```python
from build123d import *

# Parameters (mm, degrees)
SKETCH_W        = 75
SKETCH_H        = 55
PAD_DEPTH       = 3
SKETCH001_W     = 75
SKETCH001_H     = 55
SKETCH001_W_2   = 71
SKETCH001_H_2   = 51
PAD001_DEPTH    = 10
SKETCH002_W     = 5
SKETCH002_H     = 5
PAD002_DEPTH    = 5
SKETCH011_R     = 0.6
POCKET004_DEPTH = 5
SKETCH012_W     = 56
SKETCH012_H     = 10
PAD003_DEPTH    = 4
SKETCH013_W     = 8
SKETCH013_H     = 5
POCKET_DEPTH    = 8
SKETCH014_W     = 75
SKETCH014_H     = 8
PAD004_DEPTH    = 30
SKETCH015_R     = 6
PAD005_DEPTH    = 10
SKETCH016_R     = 6
PAD006_DEPTH    = 10
SKETCH017_R     = 2.2
POCKET005_DEPTH = 75
SKETCH018_W     = 55
SKETCH018_H     = 8
POCKET006_DEPTH = 8


with BuildPart() as part:
    # Sketch → Pad (new body)
    with BuildSketch(Plane.XY):
        with Locations((0, 27.5)):
            Rectangle(SKETCH_W, SKETCH_H)
    extrude(amount=PAD_DEPTH)

    # Sketch001 (on Face6 of Pad) → Pad001 (join)
    with BuildSketch(Plane.XY.offset(3)):
        with Locations((0, 27.5)):
            Rectangle(SKETCH001_W, SKETCH001_H)
        with Locations((0, 27.5)):
            Rectangle(SKETCH001_W_2, SKETCH001_H_2, mode=Mode.SUBTRACT)
    extrude(amount=PAD001_DEPTH)

    # Sketch002 (on Face15 of Pad001) → Pad002 (join)
    with BuildSketch(Plane.XY.offset(3)):
        with Locations((-33, 50.5)):
            Rectangle(SKETCH002_W, SKETCH002_H)
        with Locations((33, 50.5)):
            Rectangle(SKETCH002_W, SKETCH002_H)
        with Locations((33, 4.5)):
            Rectangle(SKETCH002_W, SKETCH002_H)
        with Locations((-33, 4.5)):
            Rectangle(SKETCH002_W, SKETCH002_H)
    extrude(amount=PAD002_DEPTH)

    # Sketch011 → Pocket004 (cut)
    with BuildSketch(Plane.XY.offset(8)):
        with Locations((-33, 4.5)):
            Circle(SKETCH011_R)
        with Locations((33, 4.5)):
            Circle(SKETCH011_R)
        with Locations((-33, 50.5)):
            Circle(SKETCH011_R)
        with Locations((33, 50.5)):
            Circle(SKETCH011_R)
    extrude(amount=-POCKET004_DEPTH, mode=Mode.SUBTRACT)

    # Sketch012 (on Face17 of Pocket004) → Pad003 (join)
    with BuildSketch(Plane.XY.offset(3)):
        with Locations((0, 33)):
            Rectangle(SKETCH012_W, SKETCH012_H)
    extrude(amount=PAD003_DEPTH)

    # Sketch013 (on Face37 of Pad003) → Pocket (cut)
    with BuildSketch(Plane.XY.offset(7)):
        with Locations((-19, 33.5)):
            Rectangle(SKETCH013_W, SKETCH013_H)
        with Locations((19, 33.5)):
            Rectangle(SKETCH013_W, SKETCH013_H)
    extrude(amount=-POCKET_DEPTH, mode=Mode.SUBTRACT)

    # Sketch014 (on Face4 of Pocket) → Pad004 (join)
    with BuildSketch(Plane(origin=(0, 0, 0), x_dir=(1, 0, 0), z_dir=(0, 0, -1))):
        with Locations((0, 4)):
            Rectangle(SKETCH014_W, SKETCH014_H)
    extrude(amount=-PAD004_DEPTH)

    # Sketch015 (on Face6 of Pad004) → Pad005 (join)
    with BuildSketch(Plane(origin=(-37.5, 0, 0), x_dir=(0, -1, 0), z_dir=(-1, 0, 0))):
        with Locations((4, 30)):
            Circle(SKETCH015_R)
    extrude(amount=-PAD005_DEPTH)

    # Sketch016 (on Face8 of Pad005) → Pad006 (join)
    with BuildSketch(Plane.YZ.offset(37.5)):
        with Locations((-4, 30)):
            Circle(SKETCH016_R)
    extrude(amount=-PAD006_DEPTH)

    # Sketch017 (on Face37 of Pad006) → Pocket005 (cut)
    with BuildSketch(Plane.YZ.offset(37.5)):
        with Locations((-4, 30)):
            Circle(SKETCH017_R)
    extrude(amount=-POCKET005_DEPTH, mode=Mode.SUBTRACT)

    # Sketch018 (on Face37 of Pocket005) → Pocket006 (cut)
    with BuildSketch(Plane.XY.offset(30)):
        with Locations((0, -4)):
            Rectangle(SKETCH018_W, SKETCH018_H)
    extrude(amount=-POCKET006_DEPTH, mode=Mode.SUBTRACT)


solid = part.part
```
Verification items for the finished model (mm, model axes). A direction names the side the tool comes from. Coordinates: 2 decimals unless noted, no trailing zeros. Write each loop counter-clockwise with the first axis right and the second up, starting at its lowest first coordinate (ties: lowest second). Pieces come first, ordered by that corner, then holes. Notation, with made-up numbers: M -19.5,-19 L -11.5,-19 A16 ccw -11.5,11 Z; hole C 54.5,-26 d5. An arc over 180 degrees is marked long. Answer as a JSON object with one key per item and string values. Group by question number.
(1) Cross-section at D-D, the plane z = 10.5. Record the cut outline in (x, y).
(2) Cross-section at C-C, the plane x = 18.5. Record the cut outline in (y, z), and give its area (3 significant figures).
(3) Cross-section at A-A, the plane z = 4.5. State how many separate pieces and enclosed holes the cut face has, and give its area (3 significant figures).
(4) Material ranges on line 1 (X direction, y = 32.5, z = 6); line 2 (Y direction, x = 13, z = 6); line 3 (Y direction, x = -33, z = 6), recorded low to high.
(5) Tool access check on faces 4 (the face through (-35.5, 27, 8)), 5 (the face through (-15, 33, 4)), 6 (the face through (-27.5, -4.1, 27.5)). Record the directions out of +Z, -Z, +X, -X, +Y, -Y that give a thin tool (end or side, any length) a straight path to the whole face; none if there is none.
(6) Cross-section at B-B, the plane y = -4. Record the cut outline in (x, z).
(7) Release check for a two-part mould opening along Y. For faces 1 (the face through (27.5, -4.1, 27.5)), 2 (the face through (33, -4, 36)), 3 (the face through (0, 28, 5)) record: +Y half, -Y half, draft (parallel to the pull), parting line (faces both ways), or undercut.
(8) Gauge pin test, flat ends, axial feed: pin 1 (6 mm diameter, centred on y = -4.5, z = 30, fed in from -X); pin 2 (2 mm diameter, centred on x = -20, z = 2, fed in from -Y); pin 3 (0.6 mm diameter, centred on x = 33, y = 4.5, fed in from +Z); pin 4 (12 mm diameter, centred on x = 9.5, z = 20.5, fed in from +Y). Record the tip position at first contact, or that the pin passes through.
Reply:
{
 "1": {"outline": "M -37.5,-8 L 37.5,-8 L 37.5,55 L -37.5,55 Z; hole M -35.5,2 L 35.5,2 L 35.5,53 L -35.5,53 Z"},
 "2": {"outline": "M -8,0 L 31,0 L 31,7 L 28,7 L 28,3 L 2,3 L 2,13 L 0,13 L 0,22 L -8,22 Z; M 36,0 L 55,0 L 55,13 L 53,13 L 53,3 L 38,3 L 38,7 L 36,7 Z", "area": "386 mm²"},
 "3": {"separate pieces": "2", "enclosed holes": "7", "area": "1,680 mm²"},
 "4": {"line 1": "-37.5 to -35.5, -28 to -23, -15 to 15, 23 to 28, 35.5 to 37.5", "line 2": "-8 to 2, 28 to 38, 53 to 55", "line 3": "-8 to 3.9, 5.1 to 7, 48 to 49.9, 51.1 to 55"},
 "5": {"face 4": "+Z", "face 5": "+Z, -Z", "face 6": "+Z, +Y, -Y"},
 "6": {"outline": "M -37.5,0 L 37.5,0 L 37.5,27.8 L 27.5,27.8 L 27.5,22 L -27.5,22 L -27.5,27.8 L -37.5,27.8 Z; M -37.5,32.2 L -27.5,32.2 L -27.5,36 L -37.5,36 Z; M 27.5,32.2 L 37.5,32.2 L 37.5,36 L 27.5,36 Z"},
 "7": {"face 1": "draft", "face 2": "parting line", "face 3": "undercut"},
 "8": {"pin 1": "x = -37.5", "pin 2": "y = -8", "pin 3": "z = 3", "pin 4": "y = 0"}
}
